Source: CAD feature listing. Evaluate the final solid. Frame: model axes, mm. Face numbers are marked on the shaded views. Coordinates: 2 decimals unless noted, no trailing zeros. Loops run counter-clockwise (first coordinate to the right, second up) from the corner with the lowest first, then second, coordinate; pieces in that order, holes last.
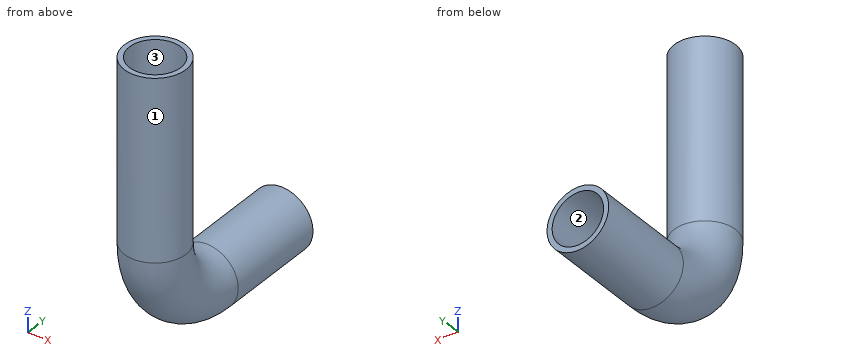
Autodesk Inventor part; units mm, degrees
ref_plane "YZ Plane" through (0, 0, 0) normal (1, 0, 0) x (0, 1, 0)
ref_plane "XZ Plane" through (0, 0, 0) normal (0, 1, 0) x (-1, 0, 0)
ref_plane "XY Plane" through (0, 0, 0) normal (0, 0, 1) x (1, 0, 0)
sketch "Sketch1" plane through (0, 0, 0) normal (0, 1, 0) x (-1, 0, 0)
  circle A0 centre (0, 0) radius 3
  circle A1 centre (0, 0) radius 2.5
  dimension "d0" = 6
  dimension "d4" = 5
sketch "Sketch2" plane through (0, 0, 0) normal (1, 0, 0) x (0, 1, 0)
  line L0 (0, 0) -> (-10, 0)
  arc A0 (-17, 7) -> (-10, 0) centre (-10, 7) ccw
  line L1 (-17, 7) -> (-17, 24.5)
  line L2 (0, -3) -> (0, 3)
  dimension "d1" = 24.5
  dimension "d2" = 7
  dimension "d3" = 17
sweep "Sweep1" add profiles "Sketch1" path "Sketch2" path curves L0 A0 L1
properties part number "24"
Q1. Section query C-C on z = 16.25. Return the cut outline in (x, y).
Q2. Draft query along Y for the marked faces 1, 2 and 3. Return one class per face: released by +Y, released by -Y, zero draft, split by the parting line, or undercut.
Q3. Section query B-B on y = -8. Return the cut outline in (x, z).
Q4. First-contact query: pin 1 Ø3 at (x, z) = (0, 0) entering from +Y; pin 2 Ø1.5 at (x, y) = (0, -17) entering from -Z. Flat tips, straight axial feed; report the tip coordinate or a pass-through.
Q5. Section query A-A on x = 0. Return the cut outline in (y, z), then the cut area to 3 significant figures.
Q6. Section query D-D on x = 2. Return the cut outline in (y, z), then the cut area to 3 significant figures.
Q7. Material intervals for line 1 along X through (y, z) = (-8, 0); line 2 along Y through (x, z) = (0, 21), sorted ascending.
Resolved:
1. outline: circle Ø6 at (0, -17); hole circle Ø5 at (0, -17)
2. face 1: split by the parting line
2. face 2: zero draft
2. face 3: undercut
3. outline: circle Ø6 at (0, 0); hole circle Ø5 at (0, 0)
4. pin 1: stops at y = -14.24
4. pin 2: stops at z = -0.81
5. outline: (-20, 7) arc R10 ccw to (-10, -3) - (0, -3) - (0, -2.5) - (-10, -2.5) arc R9.5 cw to (-19.5, 7) - (-19.5, 24.5) - (-20, 24.5) - close; (-14.5, 7) arc R4.5 ccw to (-10, 2.5) - (0, 2.5) - (0, 3) - (-10, 3) arc R4 cw to (-14, 7) - (-14, 24.5) - (-14.5, 24.5) - close
5. area: 38.5 mm2
6. outline: (-19.24, 7) arc R9.24 ccw to (-10, -2.24) - (0, -2.24) - (0, -1.5) - (-10, -1.5) arc R8.5 cw to (-18.5, 7) - (-18.5, 24.5) - (-19.24, 24.5) - close; (-15.5, 7) arc R5.5 ccw to (-10, 1.5) - (0, 1.5) - (0, 2.24) - (-10, 2.24) arc R4.76 cw to (-14.76, 7) - (-14.76, 24.5) - (-15.5, 24.5) - close
6. area: 56.7 mm2
7. line 1: x = -3 to -2.5, 2.5 to 3
7. line 2: y = -20 to -19.5, -14.5 to -14
